from build123d import *

# Parameters (mm, degrees)
FILLET1_R                = 0.5
FILLET2_R                = 1
FILLET3_R                = 1
BOSS_EXTRUDE1_DEPTH      = 1
BOSS_EXTRUDE1_DEPTH_BACK = 2


with BuildPart() as part:
    # Sketch1 → Revolve1 (revolve)
    with BuildSketch(Plane.XY):
        with BuildLine():
            Line((5.138480682, 22.4), (3.138480682, 22.4))
            Line((3.138480682, 22.4), (3.138480682, 20.4))
            Line((3.138480682, 20.4), (-10.061519318, 20.4))
            Line((-10.061519318, 20.4), (-10.061519318, 18.4))
            Line((-10.061519318, 18.4), (-3.598245279, 18.4))
            Line((-3.598245279, 18.4), (-3.598245279, 7.6))
            Line((-3.598245279, 7.6), (-10.061519318, 7.6))
            Line((-10.061519318, 7.6), (-10.061519318, 5.6))
            Line((-10.061519318, 5.6), (-3.598245279, 5.6))
            Line((-3.598245279, 5.6), (-3.598245279, 0))
            Line((-3.598245279, 0), (1.040301002, 0))
            Line((1.040301002, 0), (2.138480682, 0))
            Line((2.138480682, 0), (2.138480682, 3.907933456))
            Line((2.138480682, 3.907933456), (1.152358089, 4.47269746))
            Line((1.152358089, 4.47269746), (1.152358089, 4.972417174))
            Line((1.152358089, 4.972417174), (2.152358089, 5.472417174))
            Line((2.152358089, 5.472417174), (2.152358089, 7.972417174))
            Line((2.152358089, 7.972417174), (1.138480682, 8.5))
            Line((1.138480682, 8.5), (1.138480682, 9.5))
            Line((1.138480682, 9.5), (3.138480682, 10.5))
            Line((3.138480682, 10.5), (3.138480682, 13.5))
            Line((3.138480682, 13.5), (2.138480682, 14.5))
            Line((2.138480682, 14.5), (2.138480682, 15.5))
            Line((2.138480682, 15.5), (1.138480682, 15.5))
            Line((1.138480682, 15.5), (1.138480682, 15.9))
            Line((1.138480682, 15.9), (1.638480682, 15.9))
            Line((1.638480682, 15.9), (1.638480682, 18.4))
            Line((1.638480682, 18.4), (3.138480682, 18.4))
            ThreePointArc((3.138480682, 18.4), (4.199140854, 18.839339828), (4.638480682, 19.9))
            Line((4.638480682, 19.9), (4.638480682, 21.4))
            Line((4.638480682, 21.4), (5.138480682, 21.4))
            Line((5.138480682, 21.4), (5.138480682, 22.4))
        make_face()
    revolve(axis=Axis((-13.433569408, 0, 0), (1, 0, 0)))

    # Fillet1
    fillet1_edges = [part.edges().sort_by_distance(p)[0] for p in [
        (2.138480682, -15.5, 0),
    ]]
    fillet(fillet1_edges, radius=FILLET1_R)

    # Fillet2
    fillet2_edges = [part.edges().sort_by_distance(p)[0] for p in [
        (3.138480682, -10.5, 0),
        (3.138480682, -13.5, 0),
    ]]
    fillet(fillet2_edges, radius=FILLET2_R)

    # Fillet3
    fillet3_edges = [part.edges().sort_by_distance(p)[0] for p in [
        (2.152358089, -5.472417174, 0),
        (2.152358089, -7.972417174, 0),
    ]]
    fillet(fillet3_edges, radius=FILLET3_R)

    # Sketch2 → Boss-Extrude1 (add, two sides)
    with BuildSketch(Plane(origin=(2.138480682, 0, 0), x_dir=(0, 0, -1), z_dir=(1, 0, 0))) as boss_extrude1_sk:
        Polygon((6.997455497, 0.930333424), (8.26662156, 1.506661387), (8.402089935, 2.89395542), (7.268392248, 3.704921491), (5.999226184, 3.128593529), (5.863757809, 1.741299496), align=None)
        Polygon((1.277533, 6.942464486), (1.121606418, 8.327608276), (-0.155926582, 8.885143789), (-1.277533, 8.057535514), (-1.121606418, 6.672391724), (0.155926582, 6.114856211), align=None)
        Polygon((3.047132332, -6.367486809), (3.987446678, -7.396440329), (5.348703738, -7.096580978), (5.769646453, -5.767768106), (4.829332107, -4.738814587), (3.468075046, -5.038673938), align=None)
        Polygon((-5.114224148, -4.865656695), (-5.802243985, -6.077912906), (-5.096409229, -7.279883668), (-3.702554637, -7.26959822), (-3.0145348, -6.05734201), (-3.720369555, -4.855371247), align=None)
        Polygon((-6.207896681, 3.360345594), (-7.573430671, 3.640083573), (-8.498457863, 2.597365437), (-8.057951063, 1.274909322), (-6.692417073, 0.995171343), (-5.767389882, 2.037889479), align=None)
    extrude(amount=BOSS_EXTRUDE1_DEPTH)
    extrude(boss_extrude1_sk.sketch, amount=-BOSS_EXTRUDE1_DEPTH_BACK)


solid = part.part
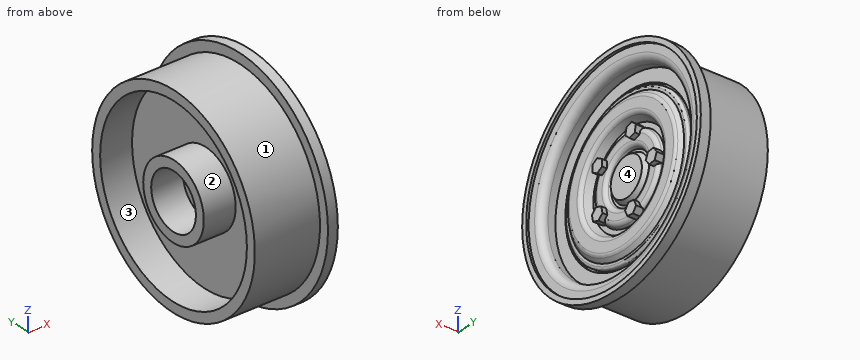
Design review of the part built by this model. Coordinates are the model's own, in mm. Face numbers are marked on the shaded views. A direction names the side the tool comes from. Coordinates: 2 decimals unless noted, no trailing zeros. Loops run counter-clockwise (first coordinate to the right, second up) from the corner with the lowest first, then second, coordinate; pieces in that order, holes last. Notation, with made-up numbers: (44.5, 40.25) -> (62.5, 40.25) arc R20 ccw to (62.5, 60.25) -> close; hole circle Ø9 at (65, -15.5). An arc over 180 degrees is marked (long way). Use a Markdown table: item, result. Add a question column.
Item 1: Clearance check with flat-ended pins moving along their axes: P1, Ø4, axis at y = 2, z = 1, coming from the +X side; P2, Ø2, axis at y = 2, z = -7, coming from the +X side; P3, Ø1.5, axis at x = -7, y = 14, coming from the -Z side. State where each tip first meets the part, or that it passes through.
Item 2: We need section A-A, the plane x = -9. Write out the cut boundary in (y, z).
Item 3: The part is to be moulded in two halves that separate along Z. For the marked faces 1 and 2, say which applies: +Z half, -Z half, draft (parallel to the pull), parting line (faces both ways), or undercut.
Item 4: Wall thickness on L1, parallel to Z at x = -6.25, y = 0; L2, parallel to Y at x = -4.5, z = -2; L3, parallel to Y at x = -8.5, z = 4: over which ranges is each line inside the solid? List them lowest first. Write a range as from..to.
Item 5: We need section B-B, the plane x = -2. Write out the cut boundary in (y, z).
Item 6: Machinability: for the marked faces 3 and 4, which of the approach directions +Z, -Z, +X, -X, +Y, -Y give a long, thin tool a straight path to every point of the face, cutting with its end or side? Answer none if there is none.
Numbers:
| question | item | result |
|---|---|---|
| 1 | P1 | stops at x = 2.14 |
| 1 | P2 | stops at x = 3.14 |
| 1 | P3 | stops at z = -15.51 |
| 2 | outline | circle Ø40.8 at (0, 0); circle Ø15.2 at (0, 0); hole circle Ø36.8 at (0, 0); hole circle Ø11.2 at (0, 0) |
| 3 | face 1 | parting line |
| 3 | face 2 | undercut |
| 4 | L1 | z = -20.4..-18.4, -7.6..-5.6, 5.6..7.6, 18.4..20.4 |
| 4 | L2 | y = -20.3..-18.29, -7.33..-5.23, 5.23..7.33, 18.29..20.3 |
| 4 | L3 | y = -20..-17.96, -6.46..-3.92, 3.92..6.46, 17.96..20 |
| 5 | outline | circle Ø40.8 at (0, 0) |
| 6 | face 3 | -X |
| 6 | face 4 | +X |
